Part print with two shaded views. Sizes in mm from the minimum x, y, z corner. A direction names the side the tool comes from. Coordinates: 2 decimals unless noted, no trailing zeros. Order: outer loops, then holes, each group sorted by start corner. A loop starts at its lowest first (then second) coordinate and runs counter-clockwise, first axis right, second up. Notation, with made-up numbers: (75, 74.5) - (96, 74.5) arc R27 ccw to (96, 96.5) - close; hole circle Ø7 at (84.25, 47.5). An arc over 180 degrees is marked (long way). One line per item, written item: value.
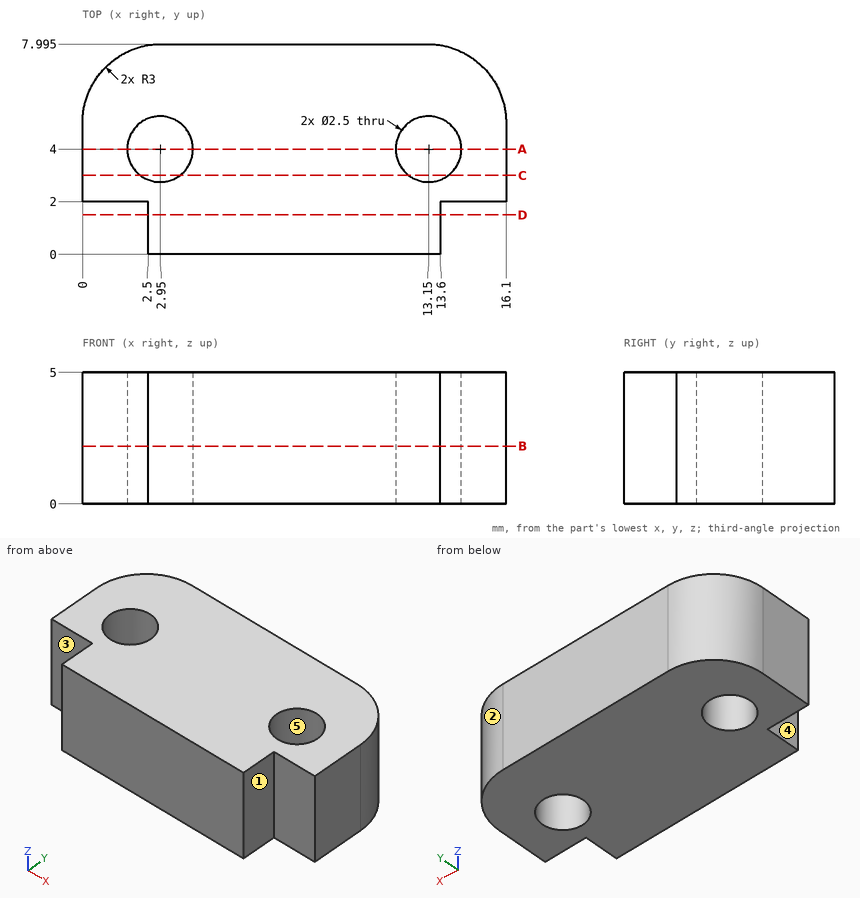
1. Probe line 1 along X through (y, z) = (4.5, 1.25) (1 decimal); line 2 along X through (y, z) = (3, 1.2); line 3 along Y through (x, z) = (13, 3.9) (1 decimal). List the from-to ranges inside material, lowest first.
Values found:
line 1: x = 0 to 1.8, 4.1 to 12, 14.3 to 16.1
line 2: x = 0 to 2.2, 3.7 to 12.4, 13.9 to 16.1
line 3: y = 0 to 2.8, 5.2 to 8
2. Band-saw the part on A-A, the plane y = 4. Give the cut face in (x, z).
Values found:
outline: (0, 0) - (1.7, 0) - (1.7, 5) - (0, 5) - close; (4.2, 0) - (11.9, 0) - (11.9, 5) - (4.2, 5) - close; (14.4, 0) - (16.1, 0) - (16.1, 5) - (14.4, 5) - close
3. 3-axis set-ups, long thin cutter, end or side, ignore diameter. For the marked faces 1 and 2: which of +Z, -Z, +X, -X, +Y, -Y reach the whole face in a straight line?
Values found:
face 1: +Z, -Z, +X, -Y
face 2: +Z, -Z, +X, +Y
4. Flat gauge pins, fed straight in: P1, Ø1.5, axis at x = 11.5, z = 1.5, coming from the -Y side; P2, Ø1.3, axis at x = 14.5, z = 3, coming from the -Y side; P3, Ø1, axis at y = 0.5, z = 2, coming from the -X side; P4, Ø1.6, axis at y = 1, z = 3.5, coming from the +X side. Where does each tip first touch, or does it go through?
Values found:
P1: stops at y = 0
P2: stops at y = 2
P3: stops at x = 2.5
P4: stops at x = 13.6
5. Band-saw the part on C-C, the plane y = 3. Give the cut face in (x, z).
Values found:
outline: (0, 0) - (2.2, 0) - (2.2, 5) - (0, 5) - close; (3.7, 0) - (12.4, 0) - (12.4, 5) - (3.7, 5) - close; (13.9, 0) - (16.1, 0) - (16.1, 5) - (13.9, 5) - close
6. Band-saw the part on D-D, the plane y = 1.5. Give the cut face in (x, z).
Values found:
outline: (2.5, 0) - (13.6, 0) - (13.6, 5) - (2.5, 5) - close
7. Band-saw the part on B-B, the plane z = 2.2. Count the separate pieces of the cut face and the enclosed holes in it, and give its area (3 significant figures).
Values found:
separate pieces: 1
enclosed holes: 2
area: 105 mm2
8. Two-plate mould, pull along Y, no slides. Class the marked faces 3, 4 and 5: pulls with the +Y half, pulls with the -Y half, needs draft (parallel to the pull), parting line crosses it, or undercut.
Values found:
face 3: pulls with the -Y half
face 4: needs draft
face 5: undercut
